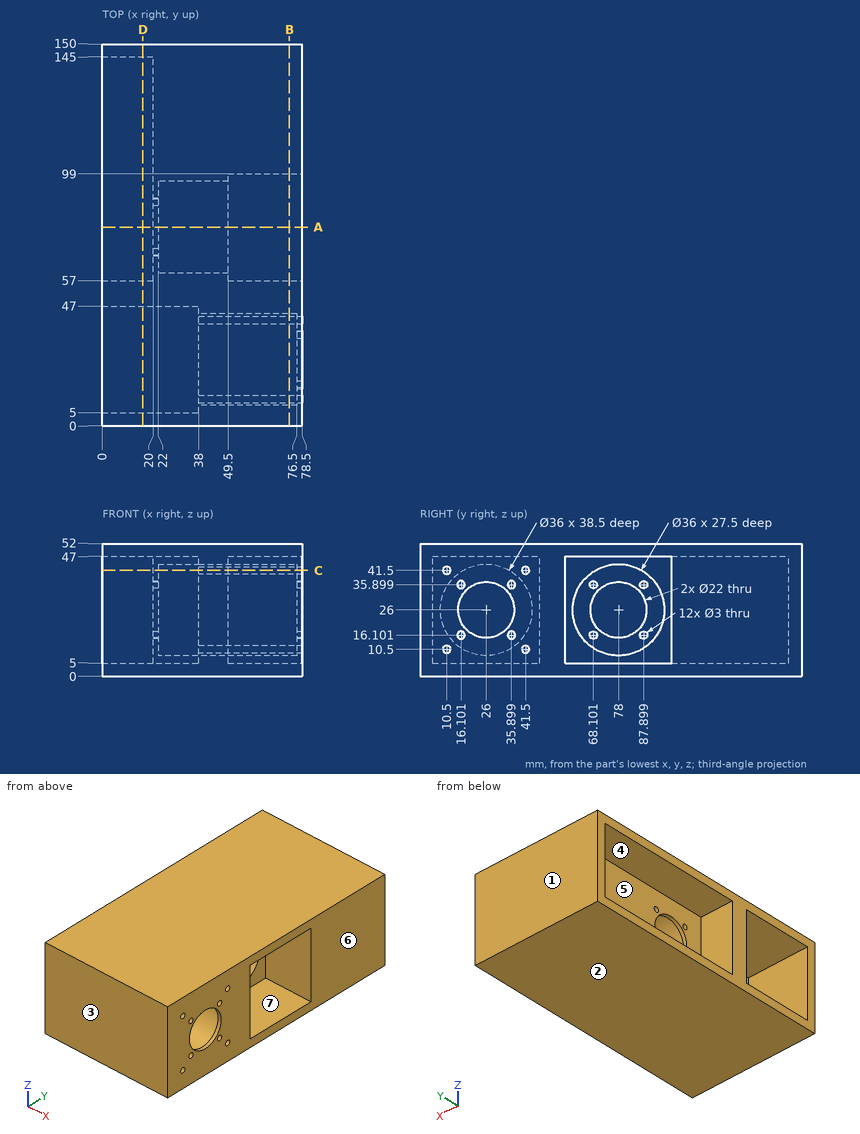
Geometry check sheet. Reference: drawing and pictorial views, mm from the part's lowest x, y, z. A direction names the side the tool comes from. Round coordinates to 2 decimals unless told otherwise and drop trailing zeros. Loops run counter-clockwise (first coordinate to the right, second up) from the corner with the lowest first, then second, coordinate; pieces in that order, holes last. Notation, with made-up numbers: (-13.75, 81.5) - (39.25, 81.5) arc R30 ccw to (39.25, 104.5) - close; hole circle Ø3 at (-32, 24.25). An arc over 180 degrees is marked (long way). Answer in a Markdown table with one row per item. Add a question column.
Q1. Gauge pin test, flat ends, axial feed: pin 1 (3.5 mm diameter, centred on y = 10.5, z = 10.5, fed in from -X); pin 2 (1 mm diameter, centred on y = 63.5, z = 30.5, fed in from -X). Record the tip position at first contact, or that the pin passes through.
Q2. Material ranges on line 1 (Y direction, x = 77.8, z = 26); line 2 (Z direction, x = 15, y = 67); line 3 (Y direction, x = 3.5, z = 31), recorded low to high.
Q3. Section check D-D on x = 16. Enter the section's corners in (y, z), plus the area to 3 significant figures.
Q4. Release check for a two-part mould opening along Y. For the marked faces 1, 2, 3 and 4 record: pulls with the +Y half, pulls with the -Y half, needs draft (parallel to the pull), parting line crosses it, or undercut.
Q5. Section check C-C on z = 41.5. State how many separate pieces and enclosed holes the cut face has, plus the area to 3 significant figures.
Q6. Section check B-B on x = 73.5. Enter the section's corners in (y, z), plus the area to 3 significant figures.
Q7. Section check A-A on y = 78. Enter the section's corners in (x, z), plus the area to 3 significant figures.
Q8. Tool access check on the marked faces 5, 6 and 7. Record the directions out of +Z, -Z, +X, -X, +Y, -Y that give a thin tool (end or side, any length) a straight path to the whole face; none if there is none.
Found:
| question | item | result |
|---|---|---|
| 1 | pin 1 | stops at x = 38 |
| 1 | pin 2 | stops at x = 20 |
| 2 | line 1 | y = 0 to 15, 37 to 57, 99 to 150 |
| 2 | line 2 | z = 0 to 5, 47 to 52 |
| 2 | line 3 | y = 0 to 5, 47 to 57, 145 to 150 |
| 3 | outline | (0, 0) - (150, 0) - (150, 52) - (0, 52) - close; hole (5, 5) - (47, 5) - (47, 47) - (5, 47) - close; hole (57, 5) - (145, 5) - (145, 47) - (57, 47) - close |
| 3 | area | 2,340 mm² |
| 4 | face 1 | pulls with the +Y half |
| 4 | face 2 | needs draft |
| 4 | face 3 | pulls with the -Y half |
| 4 | face 4 | undercut |
| 5 | separate pieces | 3 |
| 5 | enclosed holes | 0 |
| 5 | area | 5,750 mm² |
| 6 | outline | (0, 0) - (150, 0) - (150, 52) - (0, 52) - close; hole circle Ø36 at (26, 26); hole circle Ø3 at (10.5, 10.5); hole circle Ø3 at (10.5, 41.5); hole circle Ø3 at (41.5, 10.5); hole circle Ø3 at (41.5, 41.5); hole (57, 5) - (99, 5) - (99, 47) - (57, 47) - close |
| 6 | area | 4,990 mm² |
| 7 | outline | (0, 0) - (78.5, 0) - (78.5, 5) - (49.5, 5) - (49.5, 8) - (22, 8) - (22, 15) - (20, 15) - (20, 5) - (0, 5) - close; (0, 47) - (20, 47) - (20, 37) - (22, 37) - (22, 44) - (49.5, 44) - (49.5, 47) - (78.5, 47) - (78.5, 52) - (0, 52) - close |
| 7 | area | 990 mm² |
| 8 | face 5 | -X |
| 8 | face 6 | +Z, -Z, +X, +Y, -Y |
| 8 | face 7 | +X |
